Can you work these out from the drawing? Everything is in mm from the part's minimum corner. A direction names the side the tool comes from. Coordinates: 2 decimals unless noted, no trailing zeros. Order: outer loops, then holes, each group sorted by start corner. A loop starts at its lowest first (then second) coordinate and runs counter-clockwise, first axis right, second up. Notation, with made-up numbers: (-3, -5.5) -> (12, -5.5) arc R35 ccw to (12, 31.5) -> close; hole circle Ø9 at (28, 47.5). An arc over 180 degrees is marked (long way). Use a Markdown table: item, result. Add a question column.
1) If we section it at D-D (z = 122.5): Write out the boundary of the cut face in (x, y), plus the area to 3 significant figures.
2) Which directions (+Z, -Z, +X, -X, +Y, -Y) give clear straight access to the entire face, cutting with the end or side of a thin tool? Please do the marked faces 1 and 2.
3) Will these pins go through, and if not, where does the flat tip stop? pin 1 Ø6 at (x, y) = (158, 7) entering from -Z; pin 2 Ø0.9 at (y, z) = (1.5, 55) entering from +X; pin 3 Ø2.5 at (x, y) = (108.5, 1.5) entering from -Z.
4) If we section it at B-B (x = 20): Write out the boundary of the cut face in (y, z), plus the area to 3 significant figures.
5) If we section it at A-A (z = 17): Write out the boundary of the cut face in (x, y).
6) If we section it at C-C (y = 24.5): Write out the boundary of the cut face in (x, z).
7) If I drill on L1, parallel to X at y = 1.75, z = 17; L2, parallel to Z at x = 20, y = 1; L3, parallel to X at y = 17.5, z = 49, over which ranges is the centre line in solid material (lowest first)? Write a range as [from, to].
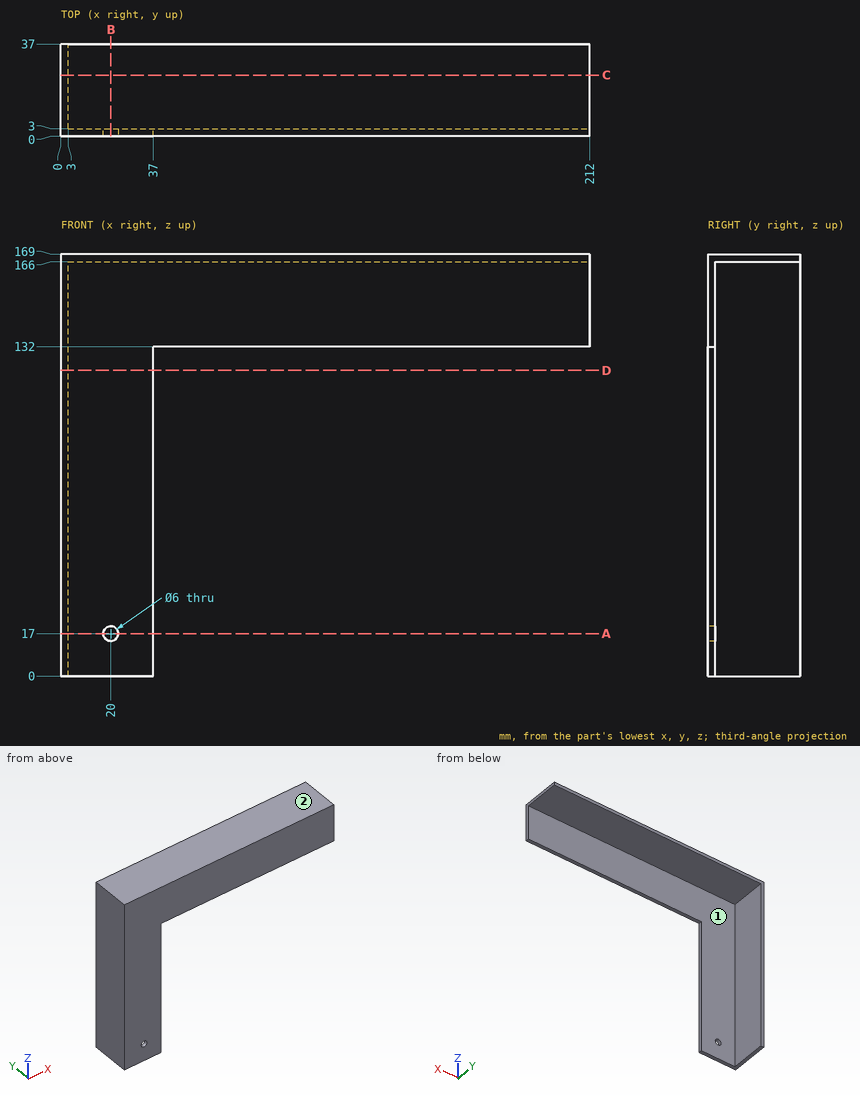
Answer sheet:
| question | item | result |
|---|---|---|
| 1 | outline | (0, 0) -> (37, 0) -> (37, 3) -> (3, 3) -> (3, 37) -> (0, 37) -> close |
| 1 | area | 213 mm2 |
| 2 | face 1 | -Z, +X, +Y |
| 2 | face 2 | +Z, +X, -X, +Y, -Y |
| 3 | pin 1 | z = 166 |
| 3 | pin 2 | x = 37 |
| 3 | pin 3 | z = 132 |
| 4 | outline | (0, 0) -> (3, 0) -> (3, 14) -> (0, 14) -> close; (0, 20) -> (3, 20) -> (3, 166) -> (37, 166) -> (37, 169) -> (0, 169) -> close |
| 4 | area | 591 mm2 |
| 5 | outline | (0, 0) -> (17, 0) -> (17, 3) -> (3, 3) -> (3, 37) -> (0, 37) -> close; (23, 0) -> (37, 0) -> (37, 3) -> (23, 3) -> close |
| 6 | outline | (0, 0) -> (3, 0) -> (3, 166) -> (212, 166) -> (212, 169) -> (0, 169) -> close |
| 7 | L1 | [0, 17], [23, 37] |
| 7 | L2 | [0, 14], [20, 169] |
| 7 | L3 | [0, 3] |
